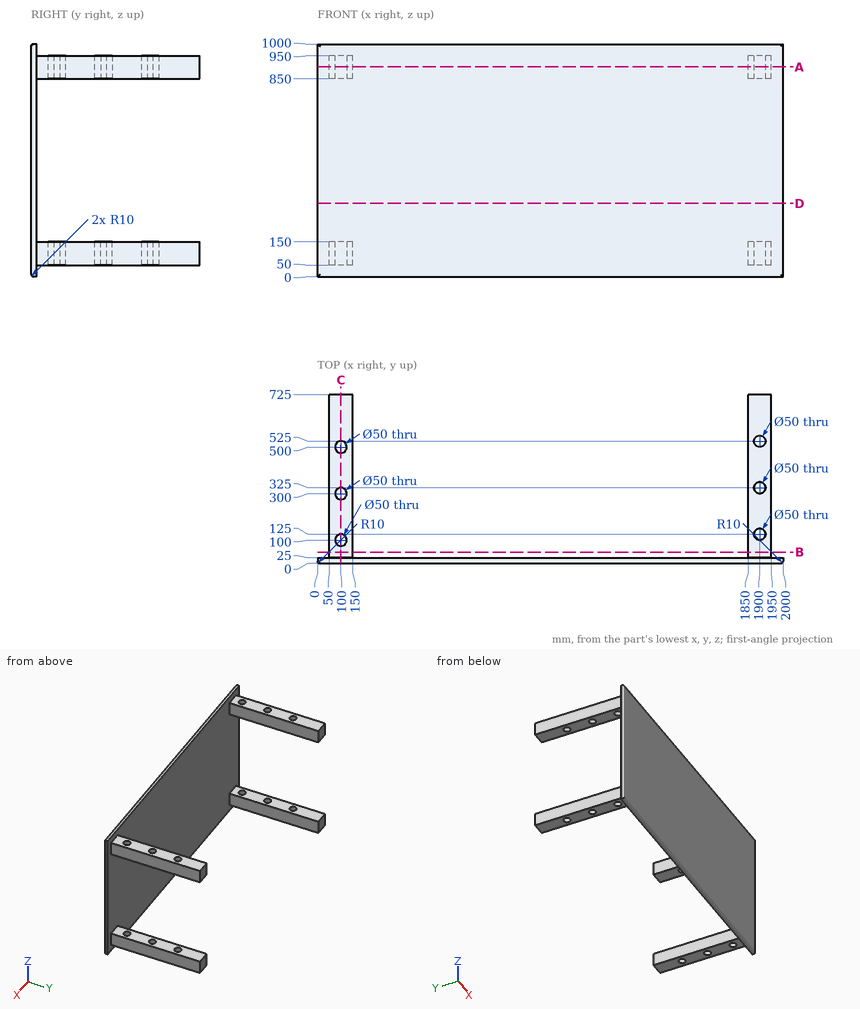
Input: dimensioned drawing with shaded views. Units: mm. Origin: part minimum x, y, z. Coordinates: 2 decimals unless noted, no trailing zeros. Loops run counter-clockwise (first coordinate to the right, second up) from the corner with the lowest first, then second, coordinate; pieces in that order, holes last. Notation, with made-up numbers: M -25,-1 L 16,-1 A25 cw 16,26 Z; hole C 53.25,-30.5 d3. An arc over 180 degrees is marked long. Use a Markdown table: item, result. Add a question column.
Q1. Section query A-A, the plane z = 902. Return loops of the section in (x, y), and give its area (3 significant figures).
Q2. Material intervals for L1, parallel to Y at x = 1900, z = 109; L2, parallel to Y at x = 100, z = 75; L3, parallel to Y at x = 1321, z = 763, sorted ascending.
Q3. Section query D-D, the plane z = 315.5. Return loops of the section in (x, y).
Q4. Section query C-C, the plane x = 100. State how many separate pieces and enclosed holes the cut face has, and give its area (3 significant figures).
Q5. Section query B-B, the plane y = 48. Return loops of the section in (x, z), and give its area (3 significant figures).
Q6. First-contact query: pin 1 (8 mm diameter, centred on y = 423, z = 105, fed in from -X); pin 2 (12 mm diameter, centred on x = 712.5, z = 393, fed in from +Y). Flat tips, straight axial feed; report the tip coordinate or a pass-through.
Result:
| question | item | result |
|---|---|---|
| 1 | outline | M 0,10 A10 ccw 10,0 L 1990,0 A10 ccw 2000,10 L 2000,25 L 1950,25 L 1950,725 L 1850,725 L 1850,25 L 150,25 L 150,725 L 50,725 L 50,25 L 0,25 Z; hole C 100,100 d50; hole C 100,300 d50; hole C 100,500 d50; hole C 1900,125 d50; hole C 1900,325 d50; hole C 1900,525 d50 |
| 1 | area | 178,000 mm2 |
| 2 | L1 | y = 0 to 100, 150 to 300, 350 to 500, 550 to 725 |
| 2 | L2 | y = 0 to 75, 125 to 275, 325 to 475, 525 to 725 |
| 2 | L3 | y = 0 to 25 |
| 3 | outline | M 0,10 A10 ccw 10,0 L 1990,0 A10 ccw 2000,10 L 2000,25 L 0,25 Z |
| 4 | separate pieces | 7 |
| 4 | enclosed holes | 0 |
| 4 | area | 135,000 mm2 |
| 5 | outline | M 50,50 L 150,50 L 150,150 L 50,150 Z; M 50,850 L 150,850 L 150,950 L 50,950 Z; M 1850,50 L 1950,50 L 1950,150 L 1850,150 Z; M 1850,850 L 1950,850 L 1950,950 L 1850,950 Z |
| 5 | area | 40,000 mm2 |
| 6 | pin 1 | stops at x = 50 |
| 6 | pin 2 | stops at y = 25 |
